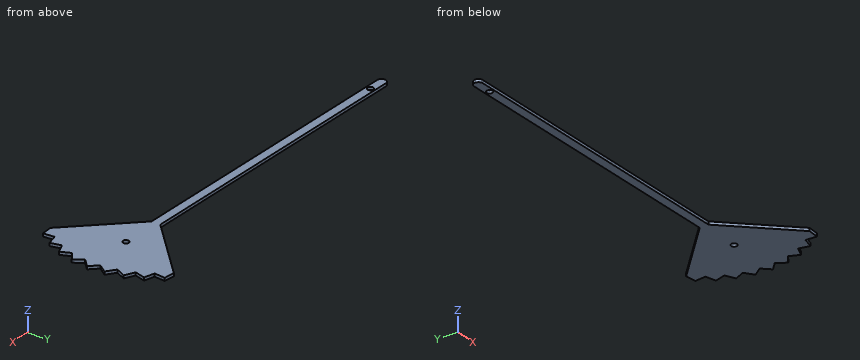
from build123d import *

# Parameters (mm, degrees)
SKETCH_1_R      = 2
EXTRUDE_1_DEPTH = 1


with BuildPart() as part:
    # 草图1 → 凸台-拉伸1 (new, symmetric)
    with BuildSketch(Plane.XY):
        with BuildLine():
            ThreePointArc((-62.732371345, 3), (-65.712136607, 0), (-62.732371345, -3))
            Line((-62.732371345, -3), (-62.69176446, -3))
            Line((-62.69176446, -3), (140.287932097, -3))
            Line((140.287932097, -3), (179.714338968, -42.426406871))
            Line((179.714338968, -42.426406871), (187.058698637, -41.880427348))
            Line((187.058698637, -41.880427348), (187.0808209, -41.78119463))
            Line((187.0808209, -41.78119463), (186.437054755, -34.414586181))
            Line((186.437054755, -34.414586181), (193.579583343, -32.5))
            Line((193.579583343, -32.5), (191.666399319, -25.357095704))
            Line((191.666399319, -25.357095704), (198.367952448, -22.231309316))
            Line((198.367952448, -22.231309316), (195.243481675, -15.529142706))
            Line((195.243481675, -15.529142706), (201.300436043, -11.287131548))
            Line((201.300436043, -11.287131548), (197.059613983, -5.229344565))
            Line((197.059613983, -5.229344565), (202.287932097, 0))
            Line((202.287932097, 0), (197.059613983, 5.229344565))
            Line((197.059613983, 5.229344565), (201.300436043, 11.287131548))
            Line((201.300436043, 11.287131548), (195.243481675, 15.529142706))
            Line((195.243481675, 15.529142706), (198.367952448, 22.231309316))
            Line((198.367952448, 22.231309316), (191.666399319, 25.357095704))
            Line((191.666399319, 25.357095704), (193.579583343, 32.5))
            Line((193.579583343, 32.5), (186.437054755, 34.414586181))
            Line((186.437054755, 34.414586181), (187.0808209, 41.78119463))
            Line((187.0808209, 41.78119463), (179.714338968, 42.426406871))
            Line((179.714338968, 42.426406871), (140.287932097, 3))
            Line((140.287932097, 3), (-62.69176446, 3))
            Line((-62.69176446, 3), (-62.732371345, 3))
        make_face()
        with Locations((-52.712067903, 0)):
            Circle(SKETCH_1_R, mode=Mode.SUBTRACT)
        with Locations((167.287932097, 0)):
            Circle(SKETCH_1_R, mode=Mode.SUBTRACT)
    extrude(amount=EXTRUDE_1_DEPTH, both=True)


solid = part.part
Read the model definition and answer for the solid it produces. Units are mm, in the model's axes. Give positions to 0.01 mm unless a question says otherwise; leave off trailing zeros. Write each loop counter-clockwise with the first axis right and the second up, starting at its lowest first coordinate (ties: lowest second). Pieces come first, ordered by that corner, then holes. Notation, with made-up numbers: (-5.75, -31) - (0.25, -31) arc R35 cw to (0.25, 7) - close; hole circle Ø11 at (8.25, 67.5). An arc over 180 degrees is marked (long way). Answer in a Markdown table with one row per item. Add a question column.
Item 1: Flat-ended cylindrical pins translate along their axes: P1, Ø5, axis at x = 167.29, y = 0, coming from the +Z side; P2, Ø1, axis at x = 86, z = 0.5, coming from the +Y side. Find the tip coordinate at first contact, or state that the pin passes through.
Item 2: Section B-B, the plane x = -16.5 is taken. Write down the section's boundary in (y, z), and give its area (3 significant figures).
Item 3: Section A-A, the plane z = -0.3 is taken. Write down the section's boundary in (x, y), and give its area (3 significant figures).
Item 4: Find the intervals of material crossed by L1, parallel to X at y = -1, z = -0.1; L2, parallel to Y at x = 54.5, z = -0.15; L3, parallel to X at y = 31, z = -0.45, in increasing order.
Recorded:
| question | item | result |
|---|---|---|
| 1 | P1 | stops at z = 1 |
| 1 | P2 | stops at y = 3 |
| 2 | outline | (-3, -1) - (3, -1) - (3, 1) - (-3, 1) - close |
| 2 | area | 12.0 mm2 |
| 3 | outline | (-62.73, -3) - (140.29, -3) - (179.71, -42.43) - (187.06, -41.88) - (187.08, -41.78) - (186.44, -34.41) - (193.58, -32.5) - (191.67, -25.36) - (198.37, -22.23) - (195.24, -15.53) - (201.3, -11.29) - (197.06, -5.23) - (202.29, 0) - (197.06, 5.23) - (201.3, 11.29) - (195.24, 15.53) - (198.37, 22.23) - (191.67, 25.36) - (193.58, 32.5) - (186.44, 34.41) - (187.08, 41.78) - (179.71, 42.43) - (140.29, 3) - (-62.73, 3) arc R3 ccw to start; hole circle Ø4 at (-52.71, 0); hole circle Ø4 at (167.29, 0) |
| 3 | area | 4,260 mm2 |
| 4 | L1 | x = -65.54 to -54.44, -50.98 to 165.56, 169.02 to 201.29 |
| 4 | L2 | y = -3 to 3 |
| 4 | L3 | x = 168.29 to 193.18 |
